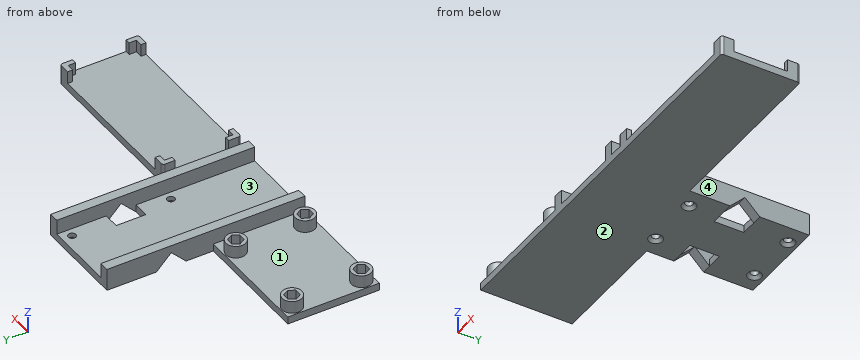
from build123d import *

# Parameters (mm, degrees)
BOSS_EXTRUDE1_START                               = 19.95
BOSS_EXTRUDE1_DEPTH                               = 4
SKETCH2_W                                         = 33
SKETCH2_H                                         = 60
BOSS_EXTRUDE2_DEPTH                               = 3
CUT_EXTRUDE1_DEPTH                                = 4
SKETCH4_W                                         = 29
SKETCH4_H                                         = 3
CUT_EXTRUDE2_DEPTH                                = 12
SKETCH5_W                                         = 22.5
SKETCH5_H                                         = 3
BOSS_EXTRUDE3_DEPTH                               = 12
BOSS_EXTRUDE4_DEPTH                               = 20
SKETCH7_W                                         = 6.5
SKETCH7_H                                         = 3
CUT_EXTRUDE3_DEPTH                                = 12
BOSS_EXTRUDE5_DEPTH                               = 4
SKETCH9_W                                         = 3
SKETCH9_H                                         = 37
BOSS_EXTRUDE6_DEPTH                               = 49
SKETCH10_W                                        = 3
SKETCH10_H                                        = 31.7
BOSS_EXTRUDE7_DEPTH                               = 72.5
CSK_FOR_M2_5_FLAT_HEAD_MACHINE_SCREW1_D           = 3.1
CSK_FOR_M2_5_FLAT_HEAD_MACHINE_SCREW1_CSINK_D     = 5.5
CSK_FOR_M2_5_FLAT_HEAD_MACHINE_SCREW1_CSINK_ANGLE = 90
BOSS_EXTRUDE8_DEPTH                               = 5
FILLET1_R                                         = 1
SKETCH26_R                                        = 4
BOSS_EXTRUDE10_DEPTH                              = 5
CUT_EXTRUDE4_DEPTH                                = 6.5


with BuildPart() as part:
    # Boss-Extrude1: read off the stored shape, not the designer's step
    # Boss-Extrude1 outline → Boss-Extrude1 (new body)
    with BuildSketch(Plane.YZ.offset(BOSS_EXTRUDE1_START)):
        Polygon((108.604346835, -99.936709039), (108.604346835, -93.936709039), (48.604346835, -93.936709039), (48.604346835, -99.936709039), (99.604346835, -99.936709039), (102.604346835, -96.936709039), (105.604346835, -99.936709039), align=None)
    extrude(amount=BOSS_EXTRUDE1_DEPTH)

    # Sketch2 → Boss-Extrude2 (add)
    with BuildSketch(Plane(origin=(0, 0, -99.936709039), x_dir=(-1, 0, 0), z_dir=(0, 0, -1))):
        with Locations((-7.45, 78.604346835)):
            Rectangle(SKETCH2_W, SKETCH2_H)
    extrude(amount=BOSS_EXTRUDE2_DEPTH)

    # Sketch3 → Cut-Extrude1 (cut)
    with BuildSketch(Plane(origin=(23.95, 0, 0), x_dir=(0, 0, -1), z_dir=(1, 0, 0))):
        Polygon((99.936709039, 99.604346835), (102.936709039, 96.604346835), (102.936709039, 108.604346835), (99.936709039, 105.604346835), align=None)
    extrude(amount=-CUT_EXTRUDE1_DEPTH, mode=Mode.SUBTRACT)

    # Sketch4 → Cut-Extrude2 (cut)
    with BuildSketch(Plane(origin=(0, 108.604346835, 0), x_dir=(-1, 0, 0), z_dir=(0, 1, 0))):
        with Locations((-5.45, -101.436709039)):
            Rectangle(SKETCH4_W, SKETCH4_H)
    extrude(amount=-CUT_EXTRUDE2_DEPTH, mode=Mode.SUBTRACT)

    # Sketch5 → Boss-Extrude3 (add)
    with BuildSketch(Plane(origin=(0, 96.604346835, 0), x_dir=(-1, 0, 0), z_dir=(0, 1, 0))):
        with Locations((-2.2, -101.436709039)):
            Rectangle(SKETCH5_W, SKETCH5_H)
    extrude(amount=BOSS_EXTRUDE3_DEPTH)

    # Sketch6 → Boss-Extrude4 (add)
    with BuildSketch(Plane(origin=(0, 108.604346835, 0), x_dir=(-1, 0, 0), z_dir=(0, 1, 0))):
        Polygon((9.05, -99.936709039), (9.05, -102.936709039), (-23.95, -102.936709039), (-23.95, -93.936709039), (-19.95, -93.936709039), (-19.95, -99.936709039), align=None)
    extrude(amount=BOSS_EXTRUDE4_DEPTH)

    # Sketch7 → Cut-Extrude3 (cut)
    with BuildSketch(Plane(origin=(0, 108.604346835, 0), x_dir=(1, 0, 0), z_dir=(0, 1, 0))):
        with Locations((-5.8, 101.436709039)):
            Rectangle(SKETCH7_W, SKETCH7_H)
    extrude(amount=-CUT_EXTRUDE3_DEPTH, mode=Mode.SUBTRACT)

    # Sketch8 → Boss-Extrude5 (add)
    with BuildSketch(Plane.ZY.offset(9.05)):
        Polygon((-102.936709039, 96.604346835), (-96.936709039, 102.604346835), (-102.936709039, 108.604346835), (-102.936709039, 128.604346835), (-93.936709039, 128.604346835), (-93.936709039, 48.604346835), (-102.936709039, 48.604346835), align=None)
    extrude(amount=BOSS_EXTRUDE5_DEPTH)

    # Sketch9 → Boss-Extrude6 (add)
    with BuildSketch(Plane.ZY.offset(13.05)):
        with Locations((-101.436709039, 67.104346835)):
            Rectangle(SKETCH9_W, SKETCH9_H)
    extrude(amount=BOSS_EXTRUDE6_DEPTH)

    # Sketch10 → Boss-Extrude7 (add)
    with BuildSketch(Plane(origin=(23.95, 0, 0), x_dir=(0, 0, -1), z_dir=(1, 0, 0))):
        with Locations((101.436709039, 64.454346835)):
            Rectangle(SKETCH10_W, SKETCH10_H)
    extrude(amount=BOSS_EXTRUDE7_DEPTH)

    # CSK for M2.5 Flat Head Machine Screw1 (through all)
    with Locations(Plane(origin=(0, 0, -102.936709039), x_dir=(-1, 0, 0), z_dir=(0, 0, -1))):
        with Locations((-16.45, 124.604346835), (-16.45, 84.604346835), (5.55, 124.604346835), (5.55, 84.604346835)):
            CounterSinkHole(CSK_FOR_M2_5_FLAT_HEAD_MACHINE_SCREW1_D / 2, CSK_FOR_M2_5_FLAT_HEAD_MACHINE_SCREW1_CSINK_D / 2, counter_sink_angle=CSK_FOR_M2_5_FLAT_HEAD_MACHINE_SCREW1_CSINK_ANGLE)

    # Sketch24 → Boss-Extrude8 (add)
    with BuildSketch(Plane.XY.offset(-99.936709039)):
        Polygon((28.95, 75.304346835), (28.95, 80.304346835), (33.95, 80.304346835), (33.95, 78.304346835), (30.95, 78.304346835), (30.95, 75.304346835), align=None)
        Polygon((91.45, 78.304346835), (91.45, 80.304346835), (96.45, 80.304346835), (96.45, 75.304346835), (94.45, 75.304346835), (94.45, 78.304346835), align=None)
        Polygon((28.95, 53.604346835), (28.95, 48.604346835), (33.95, 48.604346835), (33.95, 50.604346835), (30.95, 50.604346835), (30.95, 53.604346835), align=None)
        Polygon((96.45, 53.604346835), (96.45, 48.604346835), (91.45, 48.604346835), (91.45, 50.604346835), (94.45, 50.604346835), (94.45, 53.604346835), align=None)
    extrude(amount=BOSS_EXTRUDE8_DEPTH)

    # Fillet1
    fillet1_edges = [part.edges().sort_by_distance(p)[0] for p in [
        (96.45, 80.304346835, -98.936709039),
        (96.45, 48.604346835, -98.936709039),
        (28.95, 80.304346835, -97.436709039),
        (28.95, 48.604346835, -97.436709039),
    ]]
    fillet(fillet1_edges, radius=FILLET1_R)

    # Sketch26 → Boss-Extrude10 (add)
    with BuildSketch(Plane.XY.offset(-99.936709039)):
        with Locations(Location((-57.55, 81.104346835, 0), (0, 0, 90))):
            Circle(SKETCH26_R)
        with Locations(Location((-20.55, 81.104346835, 0), (0, 0, 90))):
            Circle(SKETCH26_R)
        with Locations(Location((-20.55, 53.104346835, 0), (0, 0, 90))):
            Circle(SKETCH26_R)
        with Locations(Location((-57.55, 53.104346835, 0), (0, 0, 90))):
            Circle(SKETCH26_R)
    extrude(amount=BOSS_EXTRUDE10_DEPTH)

    # Sketch27 → Cut-Extrude4 (cut)
    with BuildSketch(Plane.XY.offset(-94.936709039)):
        Polygon((-54.663248654, 81.104346835), (-56.106624327, 83.604346835), (-58.993375673, 83.604346835), (-60.436751346, 81.104346835), (-58.993375673, 78.604346835), (-56.106624327, 78.604346835), align=None)
        Polygon((-17.663248654, 81.104346835), (-19.106624327, 83.604346835), (-21.993375673, 83.604346835), (-23.436751346, 81.104346835), (-21.993375673, 78.604346835), (-19.106624327, 78.604346835), align=None)
        Polygon((-17.663248654, 53.104346835), (-19.106624327, 55.604346835), (-21.993375673, 55.604346835), (-23.436751346, 53.104346835), (-21.993375673, 50.604346835), (-19.106624327, 50.604346835), align=None)
        Polygon((-54.663248654, 53.104346835), (-56.106624327, 55.604346835), (-58.993375673, 55.604346835), (-60.436751346, 53.104346835), (-58.993375673, 50.604346835), (-56.106624327, 50.604346835), align=None)
    extrude(amount=-CUT_EXTRUDE4_DEPTH, mode=Mode.SUBTRACT)


solid = part.part
Input: part model. Units: mm. Frame: model coordinates. Face numbers are marked on the shaded views. A direction names the side the tool comes from. Coordinates: 2 decimals unless noted, no trailing zeros. Order: outer loops, then holes, each group sorted by start corner. A loop starts at its lowest first (then second) coordinate and runs counter-clockwise, first axis right, second up. Notation, with made-up numbers: M -0.5,-21.75 L 27.5,-21.75 A23 cw 27.5,9.25 Z; hole C 50,-33.75 d5. An arc over 180 degrees is marked long. Answer in a Markdown table with one row per item.
(1) Section query D-D, the plane y = 112. Output: boundary loops of the cut face in (x, z), plus the area to 3 significant figures.
Numbers:
| item | result |
|---|---|
| outline | M -13.05,-102.94 L 23.95,-102.94 L 23.95,-93.94 L 19.95,-93.94 L 19.95,-99.94 L -9.05,-99.94 L -9.05,-93.94 L -13.05,-93.94 Z |
| area | 159 mm^2 |
(2) Section query B-B, the plane x = -57.55. Output: boundary loops of the cut face in (y, z), plus the area to 3 significant figures.
Numbers:
| item | result |
|---|---|
| outline | M 48.6,-102.94 L 85.6,-102.94 L 85.6,-99.94 L 85.1,-99.94 L 85.1,-94.94 L 83.6,-94.94 L 83.6,-101.44 L 78.6,-101.44 L 78.6,-94.94 L 77.1,-94.94 L 77.1,-99.94 L 57.1,-99.94 L 57.1,-94.94 L 55.6,-94.94 L 55.6,-101.44 L 50.6,-101.44 L 50.6,-94.94 L 49.1,-94.94 L 49.1,-99.94 L 48.6,-99.94 Z |
| area | 126 mm^2 |
(3) Access query for the marked faces 3 and 4. Directions: +Z, -Z, +X, -X, +Y, -Y. A direction counts if a zero-diameter tool reaches every point of the face in a straight line with its end or side. Return the directions, or none.
Numbers:
| item | result |
|---|---|
| face 3 | +Z, +Y, -Y |
| face 4 | +Z, +Y |
(4) Section query A-A, the plane x = -5.55. Output: boundary loops of the cut face in (y, z), plus the area to 3 significant figures.
Numbers:
| item | result |
|---|---|
| outline | M 48.6,-102.94 L 81.85,-102.94 L 83.05,-101.74 L 83.05,-99.94 L 48.6,-99.94 Z; M 86.15,-101.74 L 87.35,-102.94 L 96.6,-102.94 L 96.6,-99.94 L 86.15,-99.94 Z; M 108.6,-102.94 L 121.85,-102.94 L 123.05,-101.74 L 123.05,-99.94 L 108.6,-99.94 Z; M 126.15,-101.74 L 127.35,-102.94 L 128.6,-102.94 L 128.6,-99.94 L 126.15,-99.94 Z |
| area | 183 mm^2 |
(5) Contact query for flat-ended pins moving along their axis: pin 1 Ø1.4 at (x, z) = (-20.5, -99.5) entering from +Y; pin 2 Ø0.6 at (x, z) = (96, -96.5) entering from +Y; pin 3 Ø4 at (x, y) = (-21, 79.5) entering from +Z; pin 4 Ø1.5 at (x, z) = (27, -96) entering from -Y. Output: stop coordinate, or through.
Numbers:
| item | result |
|---|---|
| pin 1 | stops at y = 85.6 |
| pin 2 | stops at y = 80.27 |
| pin 3 | stops at z = -94.94 |
| pin 4 | passes through |
(6) Material intervals for line 1 (Y direction, x = 16.45, z = -100.65); line 2 (X direction, y = 88, z = -99); line 3 (Y direction, x = 32, z = -95), sorted ascending. Write a range as [from, to].
Numbers:
| item | result |
|---|---|
| line 1 | y = [48.6, 83.05], [86.15, 96.6], [108.6, 123.05], [126.15, 128.6] |
| line 2 | x = [-13.05, -9.05], [19.95, 23.95] |
| line 3 | y = [48.6, 50.6], [78.3, 80.3] |
(7) Section query C-C, the plane y = 65.5. Output: boundary loops of the cut face in (x, z).
Numbers:
| item | result |
|---|---|
| outline | M -62.05,-102.94 L 96.45,-102.94 L 96.45,-99.94 L 23.95,-99.94 L 23.95,-93.94 L 19.95,-93.94 L 19.95,-99.94 L -9.05,-99.94 L -9.05,-93.94 L -13.05,-93.94 L -13.05,-99.94 L -62.05,-99.94 Z |
(8) Draft query along Y for the marked faces 1 and 2. Return one class per face: pulls with the +Y half, pulls with the -Y half, needs draft (parallel to the pull), parting line crosses it, or undercut.
Numbers:
| item | result |
|---|---|
| face 1 | undercut |
| face 2 | needs draft |
